Model file for the job. Use its own axes, mm. A direction names the side the tool comes from. Round coordinates to 2 decimals unless told otherwise and drop trailing zeros. Loops run counter-clockwise (first coordinate to the right, second up) from the corner with the lowest first, then second, coordinate; pieces in that order, holes last. Notation, with made-up numbers: M 37,-3 L 61,-3 A35 cw 61,30 Z; hole C -22,-31 d3. An arc over 180 degrees is marked long. Use a Markdown table: item, result. Add a question column.
Q1. Pin check, flat tips, straight feed: pin 1 (8 mm diameter, centred on x = 10.5, z = 13, fed in from +Y) (3 decimals); pin 2 (3 mm diameter, centred on x = 0.5, z = 5, fed in from +Y); pin 3 (2.5 mm diameter, centred on y = 5, z = 1.5, fed in from +X). Stop position of each tip, or through.
Q2. Cut at A-A (x = 5.5). Give the cut face in (y, z), plus the area to 3 significant figures.
Q3. Tool access for faces 1 (the face through (7.355, 1, 2)), 2 (the face through (-7.627, 1, 2)), 3 (the face through (0, 4.245, 17)), 4 (the face through (0, -3.285, 17)), 5 (the face through (-2, 3, 3.048)): list every direction of +Z, -Z, +X, -X, +Y, -Y with a clear straight run to the whole face (end or side of a thin tool).
Q4. Cut at B-B (y = 3.75). Give the cut face in (x, z), plus the area to 3 significant figures.
Q5. Cut at C-C (y = 0). Give the cut face in (x, z).
Q6. Mould opens along Z. For faces 6 (the face through (0, 1, 26.162)), 7 (the face through (0, 1, 0)), 8 (the face through (-2.692, -2.064, 5.427)) say: +Z half, -Z half, draft (parallel to the pull), parting line (faces both ways), or undercut.
Q7. Probe line 1 (Y direction, x = -11.5, z = 23.5); line 2 (Z direction, x = 4, y = 4.75); line 3 (Z direction, x = -11.25, y = 2.25). List the from-to ranges inside material, lowest first. Write a range as from..to.
Q8. Cut at D-D (x = 0). Give the cut face in (y, z).
from build123d import *

# Parameters (mm, degrees)
F0_W     = 14.981428
F0_H     = 15.487057
F1_DEPTH = 3.048
F2_R     = 3.391828
F3_DEPTH = 7.874
F4_W     = 26.01181
F4_H     = 7.529734
F5_DEPTH = 18.288


with BuildPart() as f1:
    # F0 (on Top) → F1 (new body)
    with BuildSketch(Plane.XY):
        with Locations((-0.136139, 1.267898)):
            Rectangle(F0_W, F0_H)
    extrude(amount=F1_DEPTH)

    # F2 (on Top) → F3 (join)
    with BuildSketch(Plane.XY):
        Circle(F2_R)
    extrude(amount=F3_DEPTH)

    # F4 (on face) → F5 (join)
    with BuildSketch(Plane.XY.offset(7.874)):
        with Locations((0.244767, 0.48016)):
            Rectangle(F4_W, F4_H)
    extrude(amount=F5_DEPTH)


solid = f1.part
Checked values:
| question | item | result |
|---|---|---|
| 1 | pin 1 | stops at y = 4.245 |
| 1 | pin 2 | stops at y = 3.39 |
| 1 | pin 3 | stops at x = 7.35 |
| 2 | outline | M -6.48,0 L 9.01,0 L 9.01,3.05 L -6.48,3.05 Z; M -3.28,7.87 L 4.25,7.87 L 4.25,26.16 L -3.28,26.16 Z |
| 2 | area | 185 mm^2 |
| 3 | face 1 | -Z, +X, +Y, -Y |
| 3 | face 2 | -Z, -X, +Y, -Y |
| 3 | face 3 | +Z, +X, -X, +Y |
| 3 | face 4 | +Z, +X, -X, -Y |
| 3 | face 5 | none |
| 4 | outline | M -12.76,7.87 L 13.25,7.87 L 13.25,26.16 L -12.76,26.16 Z; M -7.63,0 L 7.35,0 L 7.35,3.05 L -7.63,3.05 Z |
| 4 | area | 521 mm^2 |
| 5 | outline | M -12.76,7.87 L -3.39,7.87 L -3.39,3.05 L -7.63,3.05 L -7.63,0 L 7.35,0 L 7.35,3.05 L 3.39,3.05 L 3.39,7.87 L 13.25,7.87 L 13.25,26.16 L -12.76,26.16 Z |
| 6 | face 6 | +Z half |
| 6 | face 7 | -Z half |
| 6 | face 8 | undercut |
| 7 | line 1 | y = -3.28..4.25 |
| 7 | line 2 | z = 0..3.05 |
| 7 | line 3 | z = 7.87..26.16 |
| 8 | outline | M -6.48,0 L 9.01,0 L 9.01,3.05 L 3.39,3.05 L 3.39,7.87 L 4.25,7.87 L 4.25,26.16 L -3.28,26.16 L -3.28,7.87 L -3.39,7.87 L -3.39,3.05 L -6.48,3.05 Z |
